Work out the finished part from the listing and answer in its coordinate system (mm). A direction names the side the tool comes from. Give positions to 0.01 mm unless a question says otherwise; leave off trailing zeros. Write each loop counter-clockwise with the first axis right and the second up, starting at its lowest first coordinate (ties: lowest second). Pieces come first, ordered by that corner, then holes.
1) Determine the mould class of faces 1 (the face through (11.85, -24.08, 1.48)), 2 (the face through (39.92, -23.73, 1.48)), 3 (the face through (-41.96, -25.94, 1.48)) for opening direction X: pulls with the +X half, pulls with the -X half, needs draft (parallel to the pull), parting line crosses it, or undercut.
2) Find section C-C (y = 15.25). Determine the outline of the cut face in (x, z).
3) Straight lines are drawn through the part: probe 1 along Y at (x, z) = (15.25, 0.9); probe 2 along Y at (x, z) = (-15.25, 2.7); probe 3 along X at (y, z) = (29.5, 2). For each, find the intervals that lie inside material, in ascending order.
4) Find section D-D (z = 0.75). Count the separate pieces of the cut face and the enclosed holes in it, plus the area to 3 significant figures.
5) A tool of negligible diameter and unlimited length cuts with its end or side. For faces 4 (the face through (-28.148, -33.805, 1.479)), 5 (the face through (16.94, 17.91, 2.26)), 6 (the face through (36.973, -21.556, 1.479)), from which of +Z, -Z, +X, -X, +Y, -Y can it reach the whole face along a straight path? Write none if from no direction.
6) Find section A-A (x = 0). Determine the outline of the cut face in (y, z).
7) Find section B-B (y = 0). Determine the outline of the cut face in (x, z), plus the area to 3 significant figures.
8) Given pin 1 Ø16 at (x, y) = (0, 0) entering from +Z; pin 2 Ø5 at (x, y) = (-15.25, -15.25) entering from +Z; pin 3 Ø1 at (y, z) = (5, 1) entering from +X, each flat-ended and moving along its own axis, determine where each tip first touches the part or whether it passes through.
```python
from build123d import *

# Parameters (mm, degrees)
SKETCH2_R                      = 10.000000005
BOSS_EXTRUDE1_DEPTH            = 3
CBORE_FOR_M4_SHCS1_D           = 4.5
CBORE_FOR_M4_SHCS1_DEPTH       = 3
CBORE_FOR_M4_SHCS1_CBORE_D     = 6.3
CBORE_FOR_M4_SHCS1_CBORE_DEPTH = 1.5


with BuildPart() as part:
    # Sketch2 → Boss-Extrude1 (new body)
    with BuildSketch(Plane.XY):
        with BuildLine():
            Line((-13.450392883, 25.031130473), (-10.20502672, 23.105662299))
            ThreePointArc((-10.20502672, 23.105662299), (-3.968e-06, 20.306168967), (10.205019894, 23.105658249))
            Line((10.205019894, 23.105658249), (13.450387996, 25.031127573))
            ThreePointArc((13.450387996, 25.031127573), (14.094139601, 25.275272827), (14.782538902, 25.286649864))
            ThreePointArc((14.782538902, 25.286649864), (16.78075793, 25.669928952), (18.074867487, 27.239980734))
            ThreePointArc((18.074867487, 27.239980734), (18.414792088, 27.838704748), (18.937607191, 28.286681921))
            Line((18.937607191, 28.286681921), (26.321935247, 32.667786531))
            ThreePointArc((26.321935247, 32.667786531), (28.173342154, 33.821556246), (29.972660204, 35.054985063))
            Line((29.972660204, 35.054985063), (32.400972322, 36.798655128))
            ThreePointArc((32.400972322, 36.798655128), (33.891380916, 37.14769377), (35.19206653, 36.340623337))
            Line((35.19206653, 36.340623337), (41.607988179, 27.405526841))
            ThreePointArc((41.607988179, 27.405526841), (41.957026821, 25.915118247), (41.149956388, 24.614432633))
            Line((41.149956388, 24.614432633), (38.721644271, 22.870762568))
            ThreePointArc((38.721644271, 22.870762568), (36.996358641, 21.574581735), (35.32860836, 20.205164245))
            Line((35.32860836, 20.205164245), (25.926777876, 12.123874069))
            ThreePointArc((25.926777876, 12.123874069), (20.367651625, -0.007528621), (25.938200134, -12.133690637))
            Line((25.938200134, -12.133690637), (35.328603735, -20.2051589))
            ThreePointArc((35.328603735, -20.2051589), (36.996354051, -21.574576424), (38.72163972, -22.870757287))
            Line((38.72163972, -22.870757287), (41.149951774, -24.614427306))
            ThreePointArc((41.149951774, -24.614427306), (41.957022207, -25.915112921), (41.607983565, -27.405521515))
            Line((41.607983565, -27.405521515), (35.192061916, -36.340618011))
            ThreePointArc((35.192061916, -36.340618011), (33.891376301, -37.147688443), (32.400967708, -36.798649801))
            Line((32.400967708, -36.798649801), (29.97265559, -35.054979737))
            ThreePointArc((29.97265559, -35.054979737), (28.17333754, -33.82155092), (26.321930633, -32.667781205))
            Line((26.321930633, -32.667781205), (18.937602577, -28.286676595))
            ThreePointArc((18.937602577, -28.286676595), (18.414787474, -27.838699422), (18.074862873, -27.239975407))
            ThreePointArc((18.074862873, -27.239975407), (16.780753316, -25.669923625), (14.782534288, -25.286644538))
            ThreePointArc((14.782534288, -25.286644538), (14.094137778, -25.275268036), (13.450388269, -25.031125147))
            Line((13.450388269, -25.031125147), (10.205810688, -23.106124837))
            ThreePointArc((10.205810688, -23.106124837), (0.000458475, -20.306166365), (-10.205022095, -23.105656954))
            Line((-10.205022095, -23.105656954), (-13.450388259, -25.031125129))
            ThreePointArc((-13.450388259, -25.031125129), (-14.094137767, -25.275268018), (-14.782534277, -25.28664452))
            ThreePointArc((-14.782534277, -25.28664452), (-16.780753305, -25.669923607), (-18.074862862, -27.239975389))
            ThreePointArc((-18.074862862, -27.239975389), (-18.414787463, -27.838699404), (-18.937602566, -28.286676577))
            Line((-18.937602566, -28.286676577), (-26.321930622, -32.667781187))
            ThreePointArc((-26.321930622, -32.667781187), (-28.173337529, -33.821550902), (-29.972655579, -35.054979718))
            Line((-29.972655579, -35.054979718), (-32.400967697, -36.798649783))
            ThreePointArc((-32.400967697, -36.798649783), (-33.891376291, -37.147688425), (-35.192061905, -36.340617993))
            Line((-35.192061905, -36.340617993), (-41.607983554, -27.405521497))
            ThreePointArc((-41.607983554, -27.405521497), (-41.957022196, -25.915112903), (-41.149951763, -24.614427288))
            Line((-41.149951763, -24.614427288), (-38.721639646, -22.870757224))
            ThreePointArc((-38.721639646, -22.870757224), (-36.996358678, -21.574576229), (-35.328612964, -20.2051589))
            Line((-35.328612964, -20.2051589), (-25.938209362, -12.133690637))
            ThreePointArc((-25.938209362, -12.133690637), (-20.367660853, -0.007528621), (-25.926787105, 12.123874069))
            Line((-25.926787105, 12.123874069), (-35.328617589, 20.205164245))
            ThreePointArc((-35.328617589, 20.205164245), (-36.996363303, 21.574581573), (-38.721644271, 22.870762568))
            Line((-38.721644271, 22.870762568), (-41.149956388, 24.614432633))
            ThreePointArc((-41.149956388, 24.614432633), (-41.957026821, 25.915118247), (-41.607988179, 27.405526841))
            Line((-41.607988179, 27.405526841), (-35.19206653, 36.340623337))
            ThreePointArc((-35.19206653, 36.340623337), (-33.891380916, 37.14769377), (-32.400972322, 36.798655128))
            Line((-32.400972322, 36.798655128), (-29.972660204, 35.054985063))
            ThreePointArc((-29.972660204, 35.054985063), (-28.173342154, 33.821556246), (-26.321935247, 32.667786531))
            Line((-26.321935247, 32.667786531), (-18.937607191, 28.286681921))
            ThreePointArc((-18.937607191, 28.286681921), (-18.414792088, 27.838704748), (-18.074867487, 27.239980734))
            ThreePointArc((-18.074867487, 27.239980734), (-16.78075793, 25.669928952), (-14.782538902, 25.286649864))
            ThreePointArc((-14.782538902, 25.286649864), (-14.094142392, 25.275273362), (-13.450392883, 25.031130473))
        make_face()
        Circle(SKETCH2_R, mode=Mode.SUBTRACT)
    extrude(amount=BOSS_EXTRUDE1_DEPTH)

    # CBORE for M4 SHCS1
    with Locations(Plane.XY.offset(3)):
        with Locations((-32.307911482, 27.498577675), (-15.249999989, 15.249999982), (-15.249999998, -15.250000005), (-32.307911482, -27.498577711), (15.249999989, 15.249999982), (32.307911482, 27.498577675), (32.307911482, -27.498577711), (15.249999998, -15.250000005)):
            CounterBoreHole(CBORE_FOR_M4_SHCS1_D / 2, CBORE_FOR_M4_SHCS1_CBORE_D / 2, CBORE_FOR_M4_SHCS1_CBORE_DEPTH, depth=CBORE_FOR_M4_SHCS1_DEPTH)


solid = part.part
```
Results:
1. face 1: undercut
1. face 2: pulls with the +X half
1. face 3: pulls with the -X half
2. outline: (-29.56, 0) - (-17.5, 0) - (-17.5, 1.5) - (-18.4, 1.5) - (-18.4, 3) - (-29.56, 3) - close; (-13, 0) - (13, 0) - (13, 1.5) - (12.1, 1.5) - (12.1, 3) - (-12.1, 3) - (-12.1, 1.5) - (-13, 1.5) - close; (17.5, 0) - (29.56, 0) - (29.56, 3) - (18.4, 3) - (18.4, 1.5) - (17.5, 1.5) - close
3. probe 1: y = -25.25 to -17.5, -13 to 13, 17.5 to 25.25
3. probe 2: y = -25.25 to -18.4, -12.1 to 12.1, 18.4 to 25.25
3. probe 3: x = -40.1 to -34.74, -29.88 to -20.98, 20.98 to 29.88, 34.74 to 40.1
4. separate pieces: 1
4. enclosed holes: 9
4. area: 2,920 mm2
5. face 4: +Z, -Z, -Y
5. face 5: +Z
5. face 6: +Z, -Z, +X
6. outline: (-20.31, 0) - (-10, 0) - (-10, 3) - (-20.31, 3) - close; (10, 0) - (20.31, 0) - (20.31, 3) - (10, 3) - close
7. outline: (-20.37, 0) - (-10, 0) - (-10, 3) - (-20.37, 3) - close; (10, 0) - (20.37, 0) - (20.37, 3) - (10, 3) - close
7. area: 62.2 mm2
8. pin 1: passes through
8. pin 2: stops at z = 1.5
8. pin 3: stops at x = 21.34
